```python
from build123d import *

# Parameters (mm, degrees)
SKETCH_1_R          = 1.55
EXTRUDE_2_DEPTH     = 16
SKETCH_2_R          = 1.5
SKETCH_2_R_2        = 3
CUT_EXTRUDE_1_DEPTH = 25.289710071
SKETCH_3_R          = 1.5
CUT_EXTRUDE_2_DEPTH = 4


with BuildPart() as part:
    # 草图1 → 凸台-拉伸2 (new body)
    with BuildSketch(Plane.XY):
        with BuildLine():
            Line((14.20352123, 6.683160013), (-8.79647877, 6.683160013))
            Line((-8.79647877, 6.683160013), (-8.79647877, -0.066839987))
            Line((-8.79647877, -0.066839987), (-3.20121628, -0.066839987))
            ThreePointArc((-3.20121628, -0.066839987), (2.70352123, -0.816839987), (-3.20121628, -1.566839987))
            Line((-3.20121628, -1.566839987), (-8.79647877, -1.566839987))
            Line((-8.79647877, -1.566839987), (-8.79647877, -4.816839987))
            Line((-8.79647877, -4.816839987), (14.20352123, -4.816839987))
            Line((14.20352123, -4.816839987), (14.20352123, 6.683160013))
        make_face()
        with Locations((12.20352123, 0.933160013)):
            Circle(SKETCH_1_R, mode=Mode.SUBTRACT)
    extrude(amount=EXTRUDE_2_DEPTH)

    # 草图2 → 切除-拉伸1 (cut, through all)
    with BuildSketch(Plane(origin=(0, 6.683160013, 0), x_dir=(1, 0, 0), z_dir=(0, 1, 0))):
        with Locations(Location((-6.29647877, -8, 0), (0, 0, 180))):
            Circle(SKETCH_2_R)
        with Locations(Location((6.20352123, -8, 0), (0, 0, 180))):
            Circle(SKETCH_2_R_2)
    extrude(amount=-CUT_EXTRUDE_1_DEPTH, mode=Mode.SUBTRACT)

    # 草图3 → 切除-拉伸2 (cut)
    with BuildSketch(Plane.XZ.offset(4.816839987)):
        with Locations((12.20352123, 8)):
            Circle(SKETCH_3_R)
    extrude(amount=-CUT_EXTRUDE_2_DEPTH, mode=Mode.SUBTRACT)


solid = part.part
```
For this review, take the finished solid that the model builds, in its own axes (mm). A direction names the side the tool comes from. Give positions to 0.01 mm unless a question says otherwise; leave off trailing zeros. Write each loop counter-clockwise with the first axis right and the second up, starting at its lowest first coordinate (ties: lowest second). Pieces come first, ordered by that corner, then holes.
Item 1: Take a section at C-C (x = 1). Give the boundary of the cut face in (y, z).
Item 2: Take a section at A-A (z = 8). Give the boundary of the cut face in (x, y).
Item 3: Take a section at D-D (y = 4.5). Give the boundary of the cut face in (x, z), and give its area (3 significant figures).
Item 4: Take a section at B-B (y = -2). Give the boundary of the cut face in (x, z).
Item 5: Machinability: for faces 1 (the face through (3, 6.683, 8)), 2 (the face through (-6, -0.067, 6)), 3 (the face through (11.01, -2.84, 7.09)), which of the approach directions +Z, -Z, +X, -X, +Y, -Y give a long, thin tool a straight path to every point of the face, cutting with its end or side? Answer none if there is none.
Item 6: Wall thickness on probe 1 along Y at (x, z) = (-4.25, 3.5); probe 2 along X at (y, z) = (-2, 7); probe 3 along X at (y, z) = (1, 6.75): over which ranges is each line inside the solid? List them lowest first.
Item 7: Insertion check: P1, Ø3.5, axis at x = -0.3, y = -0.82, coming from the +Z side. The pin has a flat end and moves straight along its axis. Give the tip position at first contact, or say it passes through.
Item 8: The part is to be moulded in two halves that separate along Y. For faces 4 (the face through (-5.971, -3.169, 6.536)), 5 (the face through (3, -4.817, 8)), 6 (the face through (10.655, 1.001, 7.888)), say which applies: +Y half, -Y half, draft (parallel to the pull), parting line (faces both ways), or undercut.
Established:
1. outline: (-4.82, 0) - (-3.52, 0) - (-3.52, 16) - (-4.82, 16) - close; (1.89, 0) - (6.68, 0) - (6.68, 16) - (1.89, 16) - close
2. outline: (-8.8, -4.82) - (-7.8, -4.82) - (-7.8, -1.57) - (-8.8, -1.57) - close; (-8.8, -0.07) - (-7.8, -0.07) - (-7.8, 6.68) - (-8.8, 6.68) - close; (-4.8, -4.82) - (3.2, -4.82) - (3.2, 6.68) - (-4.8, 6.68) - (-4.8, -0.07) - (-3.2, -0.07) arc R3 cw (long way) to (-3.2, -1.57) - (-4.8, -1.57) - close; (9.2, -4.82) - (10.7, -4.82) - (10.7, -0.82) - (13.7, -0.82) - (13.7, -4.82) - (14.2, -4.82) - (14.2, 6.68) - (9.2, 6.68) - close; hole circle Ø3.1 at (12.2, 0.93)
3. outline: (-8.8, 0) - (14.2, 0) - (14.2, 16) - (-8.8, 16) - close; hole circle Ø3 at (-6.3, 8); hole circle Ø6 at (6.2, 8)
3. area: 333 mm2
4. outline: (-8.8, 0) - (-3.05, 0) - (-3.05, 16) - (-8.8, 16) - close; (2.46, 0) - (14.2, 0) - (14.2, 16) - (2.46, 16) - close; hole circle Ø3 at (-6.3, 8); hole circle Ø6 at (6.2, 8); hole circle Ø3 at (12.2, 8)
5. face 1: +Z, -Z, +X, -X, +Y
5. face 2: +Z, -Z, -X
5. face 3: -Y
6. probe 1: y = -4.82 to -1.57, -0.07 to 6.68
6. probe 2: x = -8.8 to -7.41, -5.18 to -3.05, 2.46 to 3.38, 9.03 to 11.09, 13.32 to 14.2
6. probe 3: x = -8.8 to -7.13, -5.47 to -2.68, 2.09 to 3.48, 8.93 to 10.65, 13.75 to 14.2
7. P1: passes through
8. face 4: draft
8. face 5: -Y half
8. face 6: undercut
